Verification items for the finished model (mm, model axes). Face numbers are marked on the shaded views. Give positions to 0.01 mm unless a question says otherwise; leave off trailing zeros.
(1) Sectioned sample at C-C on z = -13. Count the separate pieces of the cut face and the enclosed holes in it, plus the area to 3 significant figures.
(2) Gauge pin test, flat ends, axial feed: pin 1 (3 mm diameter, centred on y = 31, z = -4, fed in from +X); pin 2 (4 mm diameter, centred on x = 26, z = -5, fed in from -Y); pin 3 (2 mm diameter, centred on x = 62, z = -15, fed in from +Y). Record the tip position at first contact, or that the pin passes through.
(3) Scan lines: L1, parallel to X at y = 0, z = -14 (3 decimals); L2, parallel to X at y = 0, z = -8 (3 decimals); L3, parallel to Y at x = -51.5, z = -11. Record each from-to range of solid material in increasing order.
(4) Mould release check, pull along Y, two halves, no side actions. Record for the marked faces 1, 2 and 3: pulls with the +Y half, pulls with the -Y half, needs draft (parallel to the pull), parting line crosses it, or undercut.
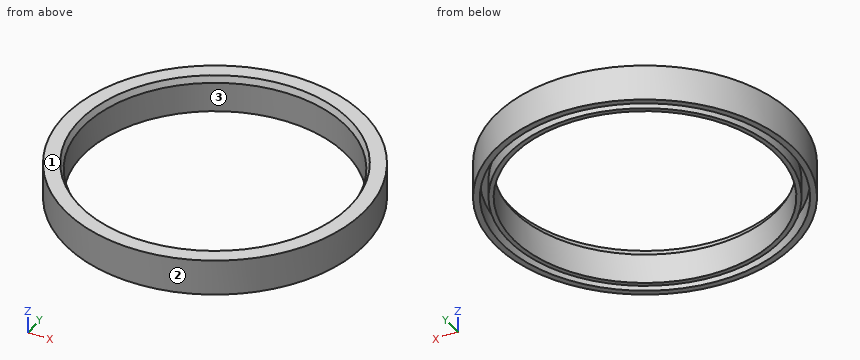
```python
from build123d import *


with BuildPart() as part:
    # Sketch2 → Revolve1 (revolve)
    with BuildSketch(Plane(origin=(0, 0, 0), x_dir=(0, 0, -1), z_dir=(1, 0, 0))):
        Polygon((0, 71.4375), (3.175, 69.85), (19.05, 69.85), (19.05, 72.23125), (9.525, 72.23125), (9.525, 76.2), (19.05, 76.2), (19.05, 79.375), (0, 79.375), align=None)
    revolve(axis=Axis((0, 0, 0), (0, 0, -1)))


solid = part.part
```
Ans:
1. separate pieces: 2
1. enclosed holes: 2
1. area: 2,610 mm2
2. pin 1: stops at x = 73.69
2. pin 2: stops at y = -75.66
2. pin 3: stops at y = 50.79
3. L1: x = -79.375 to -76.2, -72.231 to -69.85, 69.85 to 72.231, 76.2 to 79.375
3. L2: x = -79.375 to -69.85, 69.85 to 79.375
3. L3: y = -60.4 to -56.16, -50.65 to -47.19, 47.19 to 50.65, 56.16 to 60.4
4. face 1: needs draft
4. face 2: parting line crosses it
4. face 3: undercut
